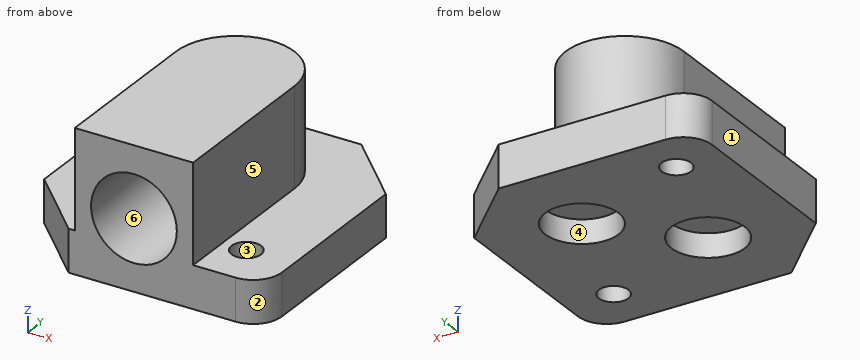
from build123d import *

# Parameters (mm, degrees)
F1_DEPTH = 9.0932
F3_DEPTH = 21.1836
F4_R     = 3.175
F5_DEPTH = 9.0942
F6_R     = 9.2075
F7_DEPTH = 28.575
F8_R     = 7.874
F9_DEPTH = 5.08


with BuildPart() as f1:
    # F0 (on Top) → F1 (new body)
    with BuildSketch(Plane.XY):
        Polygon((-27.94, 27.94), (-27.94, -14.033717), (-14.033717, -27.94), (27.94, -27.94), (27.94, 14.033717), (14.033717, 27.94), align=None)
    extrude(amount=F1_DEPTH)

    # F2 (on face) → F3 (join)
    with BuildSketch(Plane.XY.offset(9.0932)):
        with BuildLine():
            ThreePointArc((12.7, 6.985), (0, 19.685), (-12.7, 6.985))
            Line((-12.7, 6.985), (-12.7, -27.94))
            Line((-12.7, -27.94), (12.7, -27.94))
            Line((12.7, -27.94), (12.7, 6.985))
        make_face()
    extrude(amount=F3_DEPTH)

    # F4 (on face) → F5 (cut, through all)
    with BuildSketch(Plane.XY.offset(9.0932)):
        with BuildLine():
            Line((-27.94, 27.94), (-27.94, 21.799624))
            ThreePointArc((-27.94, 21.799624), (-26.141526, 26.141526), (-21.799624, 27.94))
            Line((-21.799624, 27.94), (-27.94, 27.94))
        make_face()
        with BuildLine():
            ThreePointArc((27.94, -21.799624), (26.141526, -26.141526), (21.799624, -27.94))
            Line((21.799624, -27.94), (27.94, -27.94))
            Line((27.94, -27.94), (27.94, -21.799624))
        make_face()
        with Locations((-17.843769, 17.843769)):
            Circle(F4_R)
        with Locations((17.843769, -17.843769)):
            Circle(F4_R)
    extrude(amount=-F5_DEPTH, mode=Mode.SUBTRACT)

    # F6 (on face) → F7 (cut)
    with BuildSketch(Plane.XZ.offset(27.94)):
        with Locations((0, 15.1384)):
            Circle(F6_R)
    extrude(amount=-F7_DEPTH, mode=Mode.SUBTRACT)

    # F8 (on face) → F9 (cut)
    with BuildSketch(Plane(origin=(0, 0, 0), x_dir=(1, 0, 0), z_dir=(0, 0, -1))):
        with Locations((8.351638, -8.351638)):
            Circle(F8_R)
        with Locations((-8.351638, 8.351638)):
            Circle(F8_R)
    extrude(amount=-F9_DEPTH, mode=Mode.SUBTRACT)


solid = f1.part
Check sheet for the modelled part. Datum: model origin and axes. Units: mm. Face numbers are marked on the shaded views. A direction names the side the tool comes from. Round coordinates to 2 decimals unless told otherwise and drop trailing zeros. Order: outer loops, then holes, each group sorted by start corner. A loop starts at its lowest first (then second) coordinate and runs counter-clockwise, first axis right, second up.
Q1. Cross-section at A-A, the plane x = -19.5. Enter the section's corners in (y, z).
Filled sheet:
outline: (-22.47, 0) - (15.13, 0) - (15.13, 9.09) - (-22.47, 9.09) - close; (20.55, 0) - (27.94, 0) - (27.94, 9.09) - (20.55, 9.09) - close
Q2. Draft check along X on the marked faces 1, 2 and 3. Enter one of: pulls with the +X half, pulls with the -X half, needs draft (parallel to the pull), parting line crosses it, or undercut.
Filled sheet:
face 1: pulls with the -X half
face 2: pulls with the +X half
face 3: undercut
Q3. Cross-section at C-C, the plane x = 10. Enter the section's corners in (y, z), plus the area to 3 significant figures.
Filled sheet:
outline: (-27.94, 0) - (0.65, 0) - (0.65, 5.08) - (16.05, 5.08) - (16.05, 0) - (27.94, 0) - (27.94, 9.09) - (14.81, 9.09) - (14.81, 30.28) - (-27.94, 30.28) - close
area: 1,340 mm2
Q4. Cross-section at B-B, the plane z = 11.5. Enter the section's corners in (x, y) (3 decimals), plus the area to 3 significant figures.
Filled sheet:
outline: (-12.7, -27.94) - (-8.458, -27.94) - (-8.458, 0.635) - (8.458, 0.635) - (8.458, -27.94) - (12.7, -27.94) - (12.7, 6.985) arc R12.7 ccw to (-12.7, 6.985) - close
area: 657 mm2
Q5. Depth check by flat-ended pin: P1, Ø5, axis at y = 11.5, z = 14, coming from the +X side; P2, Ø11, axis at x = 0, z = 15.14, coming from the -Y side (3 decimals); P3, Ø10, axis at y = 10, z = 19.5, coming from the +X side. Enter the tip coordinate at first touch or a pass-through.
Filled sheet:
P1: stops at x = 12.54
P2: stops at y = 0.635
P3: stops at x = 12.7
Q6. Cross-section at D-D, the plane z = 7. Enter the section's corners in (x, y) (3 decimals).
Filled sheet:
outline: (-27.94, -14.034) - (-14.034, -27.94) - (-4.306, -27.94) - (-4.306, 0.635) - (4.306, 0.635) - (4.306, -27.94) - (21.8, -27.94) arc R6.14 ccw to (27.94, -21.8) - (27.94, 14.034) - (14.034, 27.94) - (-21.8, 27.94) arc R6.14 ccw to (-27.94, 21.8) - close; hole circle Ø6.35 at (-17.844, 17.844); hole circle Ø6.35 at (17.844, -17.844)
Q7. Scan lines: L1, parallel to Z at x = 0, y = -4.75; L2, parallel to Z at x = -9, y = 17; L3, parallel to Z at x = 8, y = 13. Record each from-to range of solid material in increasing order.
Filled sheet:
L1: z = 0 to 5.93, 24.35 to 30.28
L2: z = 0 to 9.09
L3: z = 5.08 to 30.28
Q8. Set-up check for the marked faces 4, 5 and 6: record each of +Z, -Z, +X, -X, +Y, -Y from which the full face is reachable in a straight line by a thin tool's end or side.
Filled sheet:
face 4: -Z
face 5: +Z, +X, +Y, -Y
face 6: -Y
